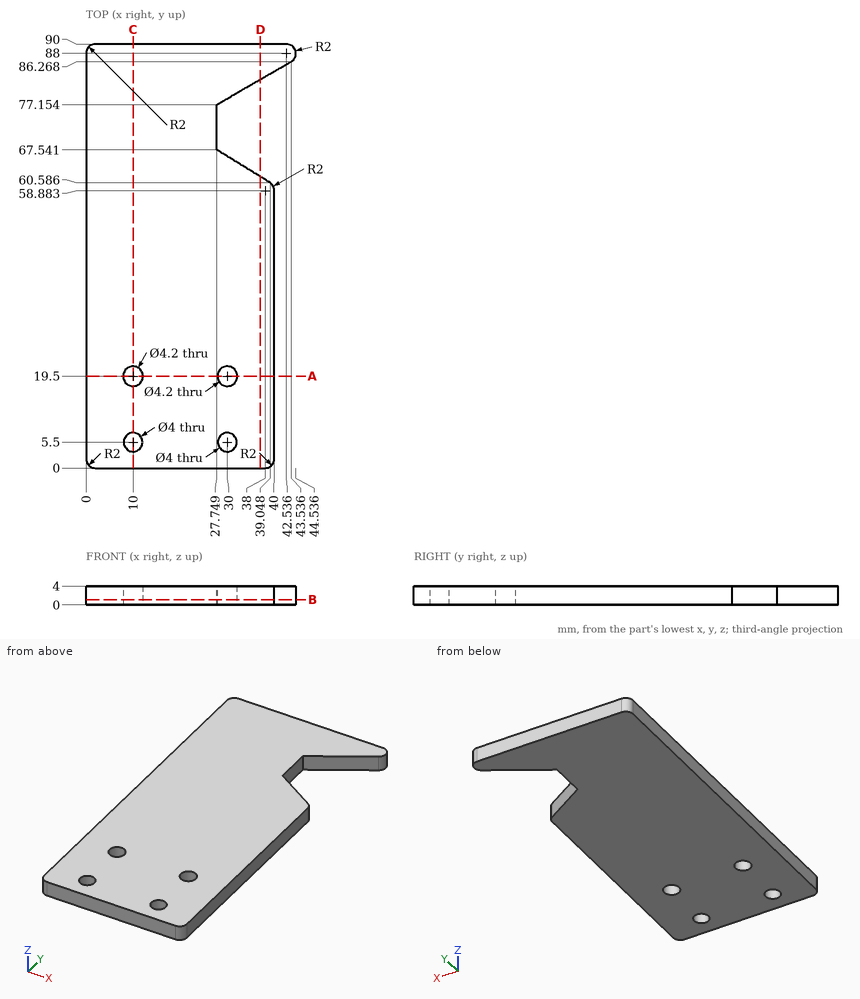
Print and shaded views of the part. All mm, measured from the part's lowest x, y and z. Give positions to 0.01 mm unless a question says otherwise; leave off trailing zeros. Order: outer loops, then holes, each group sorted by start corner. A loop starts at its lowest first (then second) coordinate and runs counter-clockwise, first axis right, second up. Notation, with made-up numbers: (-17, 68.5) - (23, 68.5) arc R26 ccw to (23, 85.5) - close; hole circle Ø10 at (81, 28). An arc over 180 degrees is marked (long way). Use a Markdown table: item, result.
1) Saw through at B-B on z = 1.15. Count the separate pieces of the cut face and the enclosed holes in it, plus the area to 3 significant figures.
Checked values:
| item | result |
|---|---|
| separate pieces | 1 |
| enclosed holes | 4 |
| area | 3,360 mm² |
2) Saw through at C-C on x = 10. List the corners of the cut face in (y, z).
Checked values:
| item | result |
|---|---|
| outline | (0, 0) - (3.5, 0) - (3.5, 4) - (0, 4) - close; (7.5, 0) - (17.4, 0) - (17.4, 4) - (7.5, 4) - close; (21.6, 0) - (90, 0) - (90, 4) - (21.6, 4) - close |
3) Probe L1, parallel to Y at x = 10, z = 2.25; L2, parallel to Y at x = 30, z = 1.55 (1 decimal); L3, parallel to Y at x = 29.5, z = 0.6 (1 decimal). List the from-to ranges inside material, lowest first. Write a range as from..to.
Checked values:
| item | result |
|---|---|
| L1 | 0..3.5, 7.5..17.4, 21.6..90 |
| L2 | 0..3.5, 7.5..17.4, 21.6..66.2, 78.5..90 |
| L3 | 0..3.6, 7.4..17.5, 21.5..66.5, 78.2..90 |
4) Flat gauge pins, fed straight in: P1, Ø4, axis at x = 10, y = 19.5, coming from the -Z side; P2, Ø1.2, axis at y = 42.5, z = 1, coming from the +X side. Where does each tip first touch, or does it go through?
Checked values:
| item | result |
|---|---|
| P1 | through |
| P2 | x = 40 |
5) Saw through at A-A on y = 19.5. List the corners of the cut face in (x, z), plus the area to 3 significant figures.
Checked values:
| item | result |
|---|---|
| outline | (0, 0) - (7.9, 0) - (7.9, 4) - (0, 4) - close; (12.1, 0) - (27.9, 0) - (27.9, 4) - (12.1, 4) - close; (32.1, 0) - (40, 0) - (40, 4) - (32.1, 4) - close |
| area | 126 mm² |
6) Saw through at D-D on x = 37. List the corners of the cut face in (y, z) (1 decimal).
Checked values:
| item | result |
|---|---|
| outline | (0, 0) - (61.8, 0) - (61.8, 4) - (0, 4) - close; (82.5, 0) - (90, 0) - (90, 4) - (82.5, 4) - close |
